```python
from build123d import *

# Parameters (mm, degrees)
BOSS_EXTRUDE1_DEPTH = 15


with BuildPart() as part:
    # Sketch1 → Boss-Extrude1 (new body)
    with BuildSketch(Plane(origin=(0, 0, 0), x_dir=(0, 0, -1), z_dir=(1, 0, 0))):
        with BuildLine():
            Line((20, 0), (66, 0))
            ThreePointArc((66, 0), (69.535533906, 1.464466094), (71, 5))
            Line((71, 5), (71, 10))
            ThreePointArc((71, 10), (72.464466094, 13.535533906), (76, 15))
            Line((76, 15), (81, 15))
            ThreePointArc((81, 15), (84.535533906, 16.464466094), (86, 20))
            Line((86, 20), (86, 66))
            ThreePointArc((86, 66), (84.535533906, 69.535533906), (81, 71))
            Line((81, 71), (76, 71))
            ThreePointArc((76, 71), (72.464466094, 72.464466094), (71, 76))
            Line((71, 76), (71, 81))
            ThreePointArc((71, 81), (69.535533906, 84.535533906), (66, 86))
            Line((66, 86), (20, 86))
            ThreePointArc((20, 86), (16.464466094, 84.535533906), (15, 81))
            Line((15, 81), (15, 76))
            ThreePointArc((15, 76), (13.535533906, 72.464466094), (10, 71))
            Line((10, 71), (5, 71))
            ThreePointArc((5, 71), (1.464466094, 69.535533906), (0, 66))
            Line((0, 66), (0, 20))
            ThreePointArc((0, 20), (1.464466094, 16.464466094), (5, 15))
            Line((5, 15), (10, 15))
            ThreePointArc((10, 15), (13.535533906, 13.535533906), (15, 10))
            Line((15, 10), (15, 5))
            ThreePointArc((15, 5), (16.464466094, 1.464466094), (20, 0))
        make_face()
    extrude(amount=BOSS_EXTRUDE1_DEPTH)


solid = part.part
```
Here's how the part is built. I have some questions about the finished solid (model axes, mm). A direction names the side the tool comes from. Give positions to 0.01 mm unless a question says otherwise; leave off trailing zeros. Loops run counter-clockwise (first coordinate to the right, second up) from the corner with the lowest first, then second, coordinate; pieces in that order, holes last. Notation, with made-up numbers: M 47.25,-25 L 57.25,-25 A37 ccw 57.25,12 Z; hole C 53,-29 d6. An arc over 180 degrees is marked long. Return JSON: item names as keys, results as strings.
Item 1: Imagine slicing it at B-B on y = 73. List the corners of the cut face in (x, z) for me, then the cut area to 3 significant figures.
A:
{"outline": "M 0,-72 L 15,-72 L 15,-14 L 0,-14 Z", "area": "870 mm^2"}
Item 2: On a 3-axis mill with a long thin cutter (end or side, diameter ignored), from which of +Z, -Z, +X, -X, +Y, -Y can I reach the whole of each face in a straight line? I mean faces 1 (the flat face through (7, 7, -71)), 2 (the flat face through (7, 79, -15)), 3 (the flat face through (7, 8, -15)), 4 (the flat face through (7, 43, 0)). Say none if no direction works.
A:
{"face 1": "-Z, +X, -X, -Y", "face 2": "+Z, +X, -X, +Y", "face 3": "+Z, +X, -X, -Y", "face 4": "+Z, +X, -X, +Y, -Y"}
Item 3: Imagine slicing it at C-C on z = -70. List the corners of the cut face in (x, y) for me, then the cut area to 3 significant figures.
A:
{"outline": "M 0,2 L 15,2 L 15,84 L 0,84 Z", "area": "1,230 mm^2"}
Item 4: Imagine slicing it at A-A on x = 2.75. List the corners of the cut face in (y, z) for me, then the cut area to 3 significant figures.
A:
{"outline": "M 0,-66 A5 ccw 5,-71 L 10,-71 A5 cw 15,-76 L 15,-81 A5 ccw 20,-86 L 66,-86 A5 ccw 71,-81 L 71,-76 A5 cw 76,-71 L 81,-71 A5 ccw 86,-66 L 86,-20 A5 ccw 81,-15 L 76,-15 A5 cw 71,-10 L 71,-5 A5 ccw 66,0 L 20,0 A5 ccw 15,-5 L 15,-10 A5 cw 10,-15 L 5,-15 A5 ccw 0,-20 Z", "area": "6,470 mm^2"}
Item 5: Please list where these lines run through material, in increasing order: line 1 (Y direction, x = 9.5, z = -77.5); line 2 (Y direction, x = 4.5, z = -69.5); line 3 (Z direction, x = 10.75, y = 4).
A:
{"line 1": "y = 15 to 71", "line 2": "y = 1.43 to 84.57", "line 3": "z = -70.9 to -15.1"}
Item 6: I'm going to push flat-ended pins straight in: pin 1 Ø5.5 at (x, z) = (9, -7) entering from +Y; pin 2 Ø5.5 at (x, y) = (8, 79) entering from -Z; pin 3 Ø2.5 at (x, z) = (9.5, -78.5) entering from -Y. Where does each tip first touch, or does it pass through?
A:
{"pin 1": "stops at y = 71", "pin 2": "stops at z = -71", "pin 3": "stops at y = 15"}
